Here's the drawing with two shaded views (mm, measured from the low corner). I have some questions. A direction names the side the tool comes from. Coordinates: 2 decimals unless noted, no trailing zeros. Write each loop counter-clockwise with the first axis right and the second up, starting at its lowest first coordinate (ties: lowest second). Pieces come first, ordered by that corner, then holes. Notation, with made-up numbers: (85.5, 52.25) -> (108.5, 52.25) arc R9 ccw to (108.5, 66.25) -> close; hole circle Ø8 at (73, -27). An arc over 180 degrees is marked (long way). Put each result on its own line as item: value. Start each with the question number.
Item 1: I want a section at D-D, the plane x = 17.75. List the corners of the cut face in (y, z) for me, then the cut area to 3 significant figures.
Item 2: I want a section at A-A, the plane z = 10.36. List the corners of the cut face in (x, y) for me (3 decimals).
Item 3: I want a section at B-B, the plane x = 10.36. List the corners of the cut face in (y, z) for me (3 decimals).
Item 4: I need wall thicknesses on line 1 (Z direction, x = 3, y = 3.4); line 2 (X direction, y = 5.2, z = 17.25); line 3 (Z direction, x = 3.5, y = 3.25). Which ranges of each line are inside material? Lowest first, please. Write a range as [from, to].
Item 5: I want a section at C-C, the plane y = 0.5. List the corners of the cut face in (x, z) for me (3 decimals).
Item 6: For pin 1 (0.9 mm diameter, centred on x = 6.985, z = 3.235, fed in from -Y); pin 2 (1.5 mm diameter, centred on y = 1, z = 8, fed in from +X); pin 3 (10 mm diameter, centred on x = 18.5, z = 15.5, fed in from -Y); pin 4 (1 mm diameter, centred on y = 3, z = 4.5, fed in from +X), each with a flat end and sliding along its axis, tell me the tip position at first contact or that it passes through.
Item 7: On a 3-axis mill with a long thin cutter (end or side, diameter ignored), from which of +Z, -Z, +X, -X, +Y, -Y can I reach the whole of each face in a straight line? I mean the marked faces 5 and 6. Say none if no direction works.
Item 8: If we mould it in two halves opening along Z, with no side actions, what happens to the marked faces 1, 2, 3 and 4? For each: released by +Z, released by -Z, zero draft, split by the parting line, or undercut.
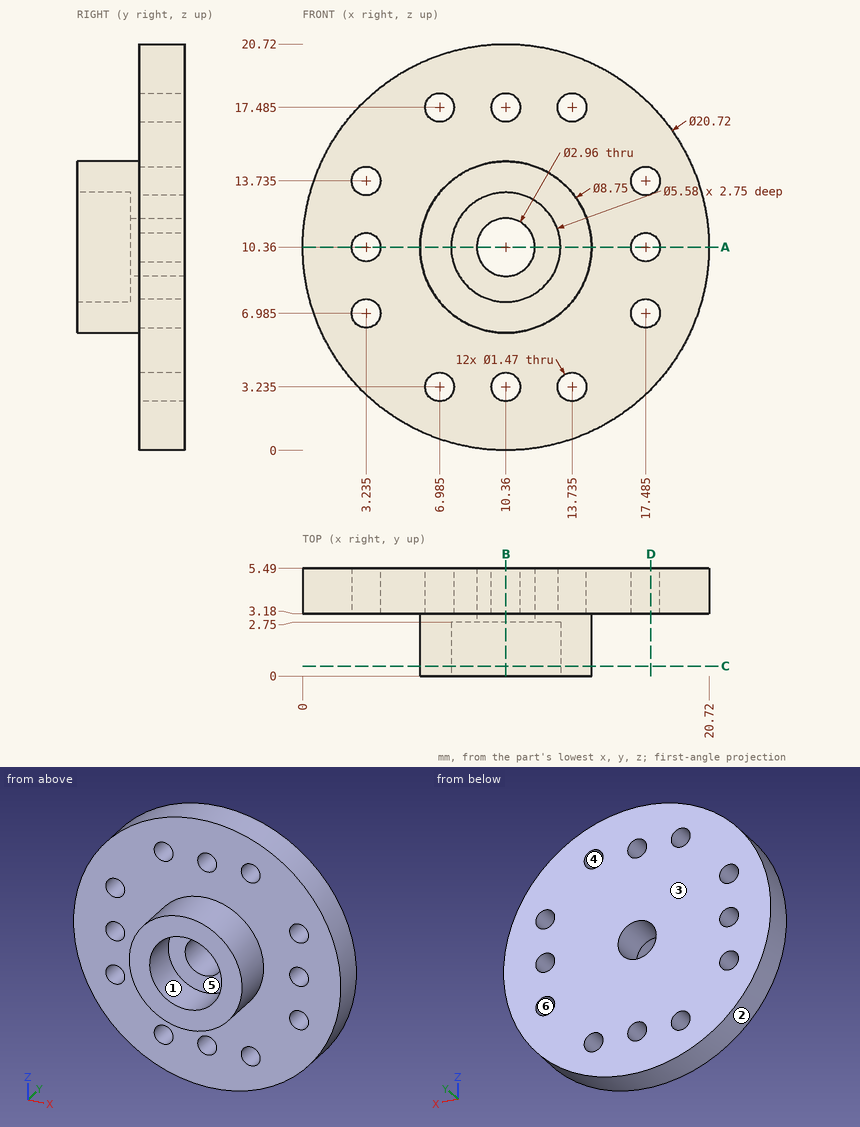
Calculated:
1. outline: (3.18, 3.1) -> (5.49, 3.1) -> (5.49, 6.3) -> (3.18, 6.3) -> close; (3.18, 7.67) -> (5.49, 7.67) -> (5.49, 9.67) -> (3.18, 9.67) -> close; (3.18, 11.05) -> (5.49, 11.05) -> (5.49, 13.05) -> (3.18, 13.05) -> close; (3.18, 14.42) -> (5.49, 14.42) -> (5.49, 17.62) -> (3.18, 17.62) -> close
1. area: 24.0 mm2
2. outline: (0, 3.18) -> (2.5, 3.18) -> (2.5, 5.49) -> (0, 5.49) -> close; (3.97, 3.18) -> (5.985, 3.18) -> (5.985, 0) -> (7.57, 0) -> (7.57, 2.75) -> (8.88, 2.75) -> (8.88, 5.49) -> (3.97, 5.49) -> close; (11.84, 2.75) -> (13.15, 2.75) -> (13.15, 0) -> (14.735, 0) -> (14.735, 3.18) -> (16.75, 3.18) -> (16.75, 5.49) -> (11.84, 5.49) -> close; (18.22, 3.18) -> (20.72, 3.18) -> (20.72, 5.49) -> (18.22, 5.49) -> close
3. outline: (0, 5.985) -> (3.18, 5.985) -> (3.18, 3.97) -> (5.49, 3.97) -> (5.49, 8.88) -> (2.75, 8.88) -> (2.75, 7.57) -> (0, 7.57) -> close; (0, 13.15) -> (2.75, 13.15) -> (2.75, 11.84) -> (5.49, 11.84) -> (5.49, 16.75) -> (3.18, 16.75) -> (3.18, 14.735) -> (0, 14.735) -> close; (3.18, 0) -> (5.49, 0) -> (5.49, 2.5) -> (3.18, 2.5) -> close; (3.18, 18.22) -> (5.49, 18.22) -> (5.49, 20.72) -> (3.18, 20.72) -> close
4. line 1: z = [3.07, 6.29], [7.68, 9.66], [11.06, 13.04], [14.43, 17.65]
4. line 2: x = [2.62, 6.29], [7.68, 9.66], [11.06, 13.04], [14.43, 18.1]
4. line 3: z = [2.6, 6.3], [7.67, 9.67], [11.05, 13.05], [14.42, 18.12]
5. outline: circle Ø8.75 at (10.36, 10.36); hole circle Ø5.58 at (10.36, 10.36)
6. pin 1: passes through
6. pin 2: stops at x = 14.43
6. pin 3: stops at y = 3.18
6. pin 4: stops at x = 19.21
7. face 5: -Y
7. face 6: +Y, -Y
8. face 1: undercut
8. face 2: split by the parting line
8. face 3: zero draft
8. face 4: undercut
